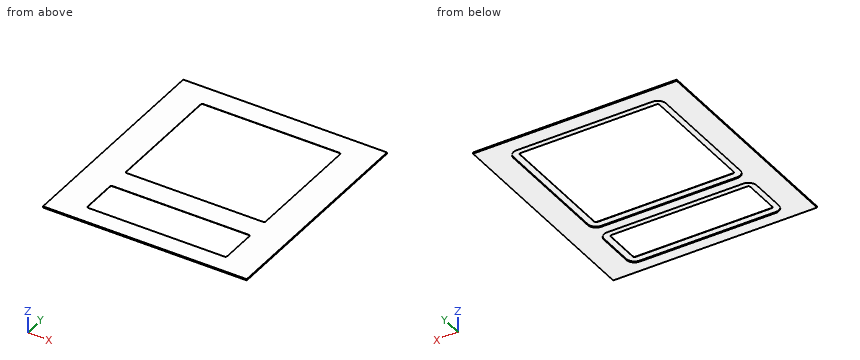
Autodesk Inventor part; units mm, degrees
ref_plane "YZ Plane" through (0, 0, 0) normal (1, 0, 0) x (0, 1, 0)
ref_plane "XZ Plane" through (0, 0, 0) normal (0, 1, 0) x (-1, 0, 0)
ref_plane "XY Plane" through (0, 0, 0) normal (0, 0, 1) x (1, 0, 0)
sketch "Sketch1" plane through (0, 0, 0) normal (0, 0, 1) x (1, 0, 0)
  line L0 (233, -255) -> (-233, -255)
  line L1 (-233, -255) -> (-233, 255)
  line L2 (-233, 255) -> (233, 255)
  line L3 (233, 255) -> (233, -255)
  line L4 (233, -255) -> (-233, 255) construction
  line L5 (-233, -255) -> (233, 255) construction
  point P0 (0, 0)
  dimension "d0" = 466
  dimension "d1" = 510
extrude "Extrusion1" add sketch "Sketch1" against normal blind 3
sketch "Sketch2" plane through (0, 0, 0) normal (0, 0, 1) x (1, 0, 0)
  line L0 (159.5, -73) -> (-159.5, -73)
  line L1 (-159.5, -73) -> (-159.5, 205)
  line L2 (-159.5, 205) -> (159.5, 205)
  line L3 (159.5, 205) -> (159.5, -73)
  line L4 (159.5, -73) -> (-159.5, 205) construction
  line L5 (-159.5, -73) -> (159.5, 205) construction
  line L6 (-233, 255) -> (-233, -255)
  line L7 (233, -255) -> (233, 255)
  line L8 (233, 255) -> (-233, 255)
  line L9 (159.5, -213) -> (-159.5, -213)
  line L10 (-159.5, -213) -> (-159.5, -125)
  line L11 (-159.5, -125) -> (159.5, -125)
  line L12 (159.5, -125) -> (159.5, -213)
  line L13 (159.5, -213) -> (-159.5, -125) construction
  line L14 (-159.5, -213) -> (159.5, -125) construction
  point P0 (0, 0)
  point P1 (0, 66)
  point P2 (0, -169)
  dimension "d4" = 73.5
  dimension "d6" = 50
  dimension "d7" = 278
  dimension "d8" = 52
  dimension "d9" = 88
extrude "Extrusion2" cut sketch "Sketch2" against normal through all
fillet "Fillet1" radius 4 8 edges at (-159.5, 205, -1.5) (159.5, 205, -1.5) (159.5, -73, -1.5) (-159.5, -73, -1.5) (-159.5, -125, -1.5) (159.5, -125, -1.5) (159.5, -213, -1.5) (-159.5, -213, -1.5)
sketch "Sketch3" plane through (0, 0, -3) normal (0, 0, -1) x (-1, 0, 0)
  line L0 (159.5, -129) -> (159.5, -209)
  arc A0 (155.5, -213) -> (159.5, -209) centre (155.5, -209) ccw
  line L1 (155.5, -213) -> (-155.5, -213)
  arc A1 (-159.5, -209) -> (-155.5, -213) centre (-155.5, -209) ccw
  line L2 (-159.5, -209) -> (-159.5, -129)
  arc A2 (-155.5, -125) -> (-159.5, -129) centre (-155.5, -129) ccw
  line L3 (-155.5, -125) -> (155.5, -125)
  arc A3 (159.5, -129) -> (155.5, -125) centre (155.5, -129) ccw
  line L4 (159.5, 201) -> (159.5, -69)
  arc A4 (155.5, -73) -> (159.5, -69) centre (155.5, -69) ccw
  line L5 (155.5, -73) -> (-155.5, -73)
  arc A5 (-159.5, -69) -> (-155.5, -73) centre (-155.5, -69) ccw
  line L6 (-159.5, -69) -> (-159.5, 201)
  arc A6 (-155.5, 205) -> (-159.5, 201) centre (-155.5, 201) ccw
  line L7 (-155.5, 205) -> (155.5, 205)
  arc A7 (159.5, 201) -> (155.5, 205) centre (155.5, 201) ccw
  line L8 (233, 255) -> (-233, 255)
  line L9 (-233, 255) -> (-233, -255)
  line L10 (-233, -255) -> (233, -255)
  line L11 (233, -255) -> (233, 255)
  line L12 (-174.5, 201) -> (-174.5, -69)
  arc A8 (-174.5, -69) -> (-155.5, -88) centre (-155.5, -69) ccw
  line L13 (-155.5, -88) -> (155.5, -88)
  arc A9 (155.5, -88) -> (174.5, -69) centre (155.5, -69) ccw
  line L14 (174.5, -69) -> (174.5, 201)
  arc A10 (174.5, 201) -> (155.5, 220) centre (155.5, 201) ccw
  line L15 (155.5, 220) -> (-155.5, 220)
  arc A11 (-155.5, 220) -> (-174.5, 201) centre (-155.5, 201) ccw
  line L16 (155.5, -110) -> (-155.5, -110)
  arc A12 (-155.5, -110) -> (-174.5, -129) centre (-155.5, -129) ccw
  line L17 (-174.5, -129) -> (-174.5, -209)
  arc A13 (-174.5, -209) -> (-155.5, -228) centre (-155.5, -209) ccw
  line L18 (-155.5, -228) -> (155.5, -228)
  arc A14 (155.5, -228) -> (174.5, -209) centre (155.5, -209) ccw
  line L19 (174.5, -209) -> (174.5, -129)
  arc A15 (174.5, -129) -> (155.5, -110) centre (155.5, -129) ccw
  point P0 (0, 0)
  dimension "d13" = 15
  dimension "d14" = 15
extrude "Extrusion3" cut sketch "Sketch3" against normal blind 2.3813 contours A11 L15 A10 L14 A9 L13 A8 L12 | A15 L19 A14 L18 A13 L17 A12 L16
properties part number "Door Panel" material "PET Plastic"
For this review, take the finished solid that the model builds, in its own axes (mm). Round coordinates to 2 decimals unless told otherwise and drop trailing zeros. Loops run counter-clockwise (first coordinate to the right, second up) from the corner with the lowest first, then second, coordinate; pieces in that order, holes last.
Q1. To check wall thickness, follow line 1 along Y through (x, z) = (73, -0.95); line 2 along Y through (x, z) = (81, -0.45); line 3 along X through (y, z) = (28.5, -1.7). State the ranges of each line that lie inside material, in increasing order.
Result sheet:
line 1: y = -255 to -228, -110 to -88, 220 to 255
line 2: y = -255 to -213, -125 to -73, 205 to 255
line 3: x = -233 to -174.5, 174.5 to 233
Q2. Add section B-B on z = -2.4. Write out the cut boundary in (x, y).
Result sheet:
outline: (-233, -255) - (233, -255) - (233, 255) - (-233, 255) - close; hole (-174.5, -209) arc R19 ccw to (-155.5, -228) - (155.5, -228) arc R19 ccw to (174.5, -209) - (174.5, -129) arc R19 ccw to (155.5, -110) - (-155.5, -110) arc R19 ccw to (-174.5, -129) - close; hole (-174.5, -69) arc R19 ccw to (-155.5, -88) - (155.5, -88) arc R19 ccw to (174.5, -69) - (174.5, 201) arc R19 ccw to (155.5, 220) - (-155.5, 220) arc R19 ccw to (-174.5, 201) - close
Q3. Add section C-C on x = 114. Write out the cut boundary in (y, z).
Result sheet:
outline: (-255, -3) - (-228, -3) - (-228, -0.62) - (-213, -0.62) - (-213, 0) - (-255, 0) - close; (-125, -0.62) - (-110, -0.62) - (-110, -3) - (-88, -3) - (-88, -0.62) - (-73, -0.62) - (-73, 0) - (-125, 0) - close; (205, -0.62) - (220, -0.62) - (220, -3) - (255, -3) - (255, 0) - (205, 0) - close
Q4. Add section A-A on y = 93. Write out the cut boundary in (x, z).
Result sheet:
outline: (-233, -3) - (-174.5, -3) - (-174.5, -0.62) - (-159.5, -0.62) - (-159.5, 0) - (-233, 0) - close; (159.5, -0.62) - (174.5, -0.62) - (174.5, -3) - (233, -3) - (233, 0) - (159.5, 0) - close
